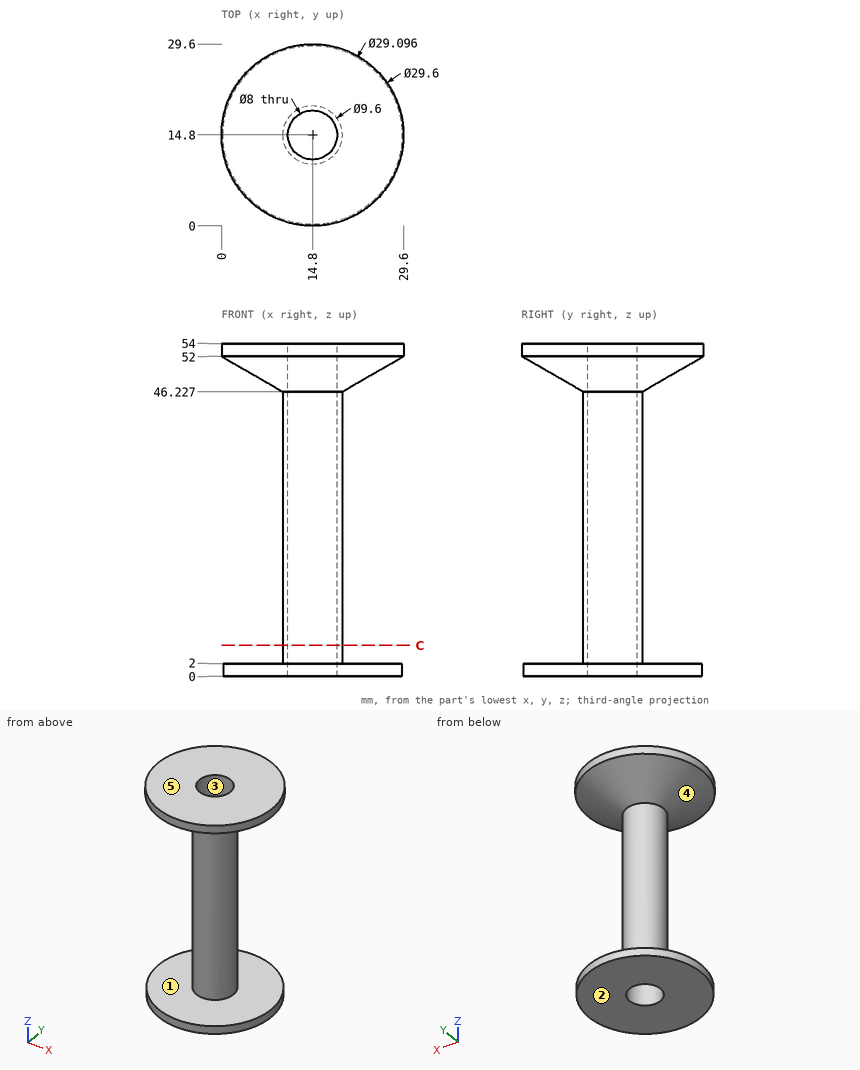
Study the drawing (mm; zero at the part's minimum x, y, z) and answer. A direction names the side the tool comes from. Give positions to 0.01 mm unless a question says otherwise; leave off trailing zeros. Write each loop counter-clockwise with the first axis right and the second up, starting at its lowest first coordinate (ties: lowest second). Pieces come first, ordered by that corner, then holes.
Item 1: Determine the mould class of the marked faces 3, 4 and 5 for opening direction X: released by +X, released by -X, zero draft, split by the parting line, or undercut.
Item 2: Find the intervals of material crossed by line 1 along Y through (x, z) = (14.8, 41); line 2 along Z through (x, y) = (25.75, 7.25) (1 decimal); line 3 along Z through (x, y) = (17, 8.75), in increasing order.
Item 3: Section C-C, the plane z = 5 is taken. Write down the section's boundary in (x, y).
Item 4: Which of the six approach directions +Z, -Z, +X, -X, +Y, -Y give full straight-line access (tool end or side, diameter ignored) to the marked faces 1 and 2?
Item 5: Flat-ended cylindrical pins translate along their axes: P1, Ø8, axis at y = 14.5, z = 29, coming from the -X side; P2, Ø1.5, axis at x = 11, z = 38.5, coming from the -Y side (1 decimal); P3, Ø1.5, axis at x = 10, z = 30, coming from the -Y side (1 decimal). Find the tip coordinate at first contact, or state that the pin passes through.
Completed:
1. face 3: undercut
1. face 4: split by the parting line
1. face 5: zero draft
2. line 1: y = 10 to 10.8, 18.8 to 19.6
2. line 2: z = 0 to 2, 51.1 to 54
2. line 3: z = 0 to 2, 47.17 to 54
3. outline: circle Ø9.6 at (14.8, 14.8); hole circle Ø8 at (14.8, 14.8)
4. face 1: none
4. face 2: -Z, +X, -X, +Y, -Y
5. P1: stops at x = 10
5. P2: stops at y = 11.1
5. P3: stops at y = 12.2
